Geometry check sheet. Reference: the model listing, model coordinates, mm. Face numbers are marked on the shaded views. A direction names the side the tool comes from. Coordinates: 2 decimals unless noted, no trailing zeros. Write each loop counter-clockwise with the first axis right and the second up, starting at its lowest first coordinate (ties: lowest second). Pieces come first, ordered by that corner, then holes. Notation, with made-up numbers: (-14.75, 82) - (-5.75, 82) arc R13 cw to (-5.75, 86) - close; hole circle Ø2 at (-39, 10). An arc over 180 degrees is marked (long way). Answer as a JSON object with one key per item and string values. Group by question number.
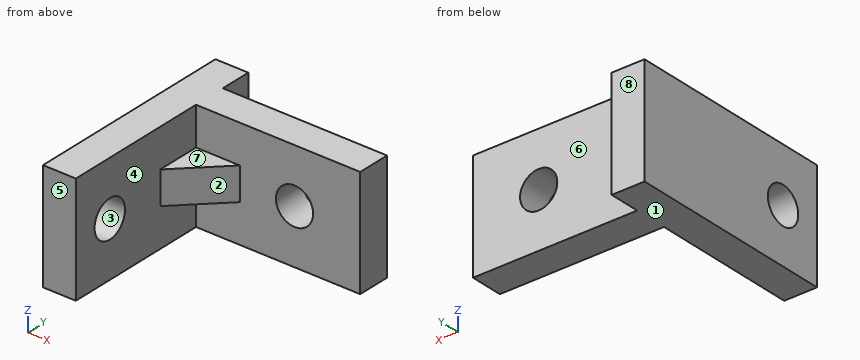
from build123d import *

# Parameters (mm, degrees)
BOSS_EXTRUDE1_DEPTH = 5
SKETCH2_R           = 1.7
CUT_EXTRUDE1_DEPTH  = 25.891815924
SKETCH3_R           = 1.7
CUT_EXTRUDE2_DEPTH  = 24.019611204
SKETCH5_W           = 3
SKETCH5_H           = 2.85
BOSS_EXTRUDE2_DEPTH = 10
BOSS_EXTRUDE3_DEPTH = 1.5


with BuildPart() as part:
    # Sketch1 → Boss-Extrude1 (new, symmetric)
    with BuildSketch(Plane.XY):
        Polygon((0, 0), (3, 0), (3, 13.45), (18, 13.45), (18, 16.45), (0, 16.45), align=None)
    extrude(amount=BOSS_EXTRUDE1_DEPTH, both=True)

    # Sketch2 → Cut-Extrude1 (cut, through all)
    with BuildSketch(Plane.ZY):
        with Locations(Location((0, 3.8, 0), (0, 0, 270))):
            Circle(SKETCH2_R)
    extrude(amount=-CUT_EXTRUDE1_DEPTH, mode=Mode.SUBTRACT)

    # Sketch3 → Cut-Extrude2 (cut, through all)
    with BuildSketch(Plane.XZ.offset(-13.45)):
        with Locations(Location((12, 0, 0), (0, 0, 270))):
            Circle(SKETCH3_R)
    extrude(amount=-CUT_EXTRUDE2_DEPTH, mode=Mode.SUBTRACT)

    # Sketch5 → Boss-Extrude2 (add)
    with BuildSketch(Plane.XY.offset(5)):
        with Locations((1.5, 17.875)):
            Rectangle(SKETCH5_W, SKETCH5_H)
    extrude(amount=-BOSS_EXTRUDE2_DEPTH)

    # Sketch6 → Boss-Extrude3 (add, symmetric)
    with BuildSketch(Plane.XY):
        Polygon((7, 13.45), (3, 9.45), (3, 13.45), align=None)
    extrude(amount=BOSS_EXTRUDE3_DEPTH, both=True)


solid = part.part
(1) Section check B-B (x = 12). Record the cut outline in (y, z), and give its area (3 significant figures).
(2) Section check A-A (y = 3.8). Record the cut outline in (x, z).
(3) Material ranges on L1, parallel to X at y = 15.25, z = 0; L2, parallel to Z at x = 2.3, y = 3.8; L3, parallel to Y at x = 5.75, z = -1.75, recorded low to high. Write a range as [from, to].
(4) Set-up check for the marked faces 4, 5, 6, 7 and 8: record each of +Z, -Z, +X, -X, +Y, -Y from which the full face is reachable in a straight line by a thin tool's end or side.
(5) Section check D-D (x = 4). Record the cut outline in (y, z).
(6) Draft check along Z on the marked faces 1, 2 and 3. Enter one of: +Z half, -Z half, draft (parallel to the pull), parting line (faces both ways), or undercut.
(7) Gauge pin test, flat ends, axial feed: pin 1 (6 mm diameter, centred on x = 15.5, z = -1.5, fed in from -Y); pin 2 (3 mm diameter, centred on y = 18, z = 1.5, fed in from +X); pin 3 (5 mm diameter, centred on y = 9, z = -1, fed in from +X); pin 4 (2 mm diameter, centred on y = 3.8, z = 0, fed in from -X). Record the tip position at first contact, or that the pin passes through.
(8) Section check C-C (z = 0). Record the cut outline in (x, y), and give its area (3 significant figures).
Conclusion:
{
 "1": {"outline": "(13.45, -5) - (16.45, -5) - (16.45, -1.7) - (13.45, -1.7) - close; (13.45, 1.7) - (16.45, 1.7) - (16.45, 5) - (13.45, 5) - close", "area": "19.8 mm^2"},
 "2": {"outline": "(0, -5) - (3, -5) - (3, -1.7) - (0, -1.7) - close; (0, 1.7) - (3, 1.7) - (3, 5) - (0, 5) - close"},
 "3": {"L1": "x = [0, 10.3], [13.7, 18]", "L2": "z = [-5, -1.7], [1.7, 5]", "L3": "y = [13.45, 16.45]"},
 "4": {"face 4": "+X, -Y", "face 5": "+Z, -Z, +X, -X, -Y", "face 6": "+Z, -Z, +X, +Y", "face 7": "+Z, +X, -Y", "face 8": "+Z, -Z, +X, -X, +Y"},
 "5": {"outline": "(10.45, -1.5) - (13.45, -1.5) - (13.45, -5) - (16.45, -5) - (16.45, 5) - (13.45, 5) - (13.45, 1.5) - (10.45, 1.5) - close"},
 "6": {"face 1": "-Z half", "face 2": "draft", "face 3": "undercut"},
 "7": {"pin 1": "stops at y = 13.45", "pin 2": "stops at x = 3", "pin 3": "stops at x = 5.05", "pin 4": "passes through"},
 "8": {"outline": "(0, 0) - (3, 0) - (3, 2.1) - (0, 2.1) - close; (0, 5.5) - (3, 5.5) - (3, 9.45) - (7, 13.45) - (10.3, 13.45) - (10.3, 16.45) - (3, 16.45) - (3, 19.3) - (0, 19.3) - close; (13.7, 13.45) - (18, 13.45) - (18, 16.45) - (13.7, 16.45) - close", "area": "90.5 mm^2"}
}
